Autodesk Inventor part; units mm, degrees
ref_plane "YZ Plane" through (0, 0, 0) normal (1, 0, 0) x (0, 1, 0)
ref_plane "XZ Plane" through (0, 0, 0) normal (0, 1, 0) x (-1, 0, 0)
ref_plane "XY Plane" through (0, 0, 0) normal (0, 0, 1) x (1, 0, 0)
sketch "Sketch1" plane through (0, 0, 0) normal (0, 0, 1) x (1, 0, 0)
  line L0 (-7.5896, 2.5423) -> (-6.4349, 4.5423)
  line L1 (-6.4349, 4.5423) -> (-4.1255, 4.5423)
  line L2 (-4.1255, 4.5423) -> (-2.9708, 2.5423)
  line L3 (-2.9708, 2.5423) -> (-4.1255, 0.5423)
  line L4 (-4.1255, 0.5423) -> (-6.4349, 0.5423)
  line L5 (-6.4349, 0.5423) -> (-7.5896, 2.5423)
  circle A0 centre (-5.2802, 2.5423) radius 1
  dimension "d0" = 4
  dimension "d1" = 2
extrude "Extrusion1" add sketch "Sketch1" along normal blind 10 contours L0 L1 L2 L3 L4 L5 | A0
extrude "Extrusion2" add sketch "Sketch1" against normal blind 6 contours A0
sketch "Sketch2" plane through (0, 0, 10) normal (0, 0, 1) x (1, 0, 0)
  circle A0 centre (-5.2802, 2.5423) radius 1
  circle A1 centre (-5.2802, 2.5423) radius 1.5
  point P0 (0, 0)
hole "Hole1" at (-5.2802, 2.5423, 10) direction (0, 0, -1) diameter 2 depth 7 tip angle 120
chamfer "Chamfer1" distance 0.1 angle 45 1 edges at (-6.2802, 2.5423, -6)
thread "Thread3"
thread "Thread4"
properties part number "Espaciador de Plástico M2 L10" material "Brass, Soft Yellow"
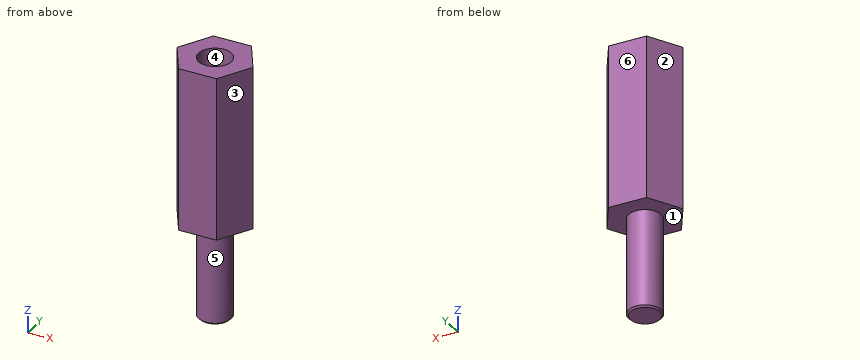
Input: part model. Units: mm. Frame: model coordinates. Face numbers are marked on the shaded views. A direction names the side the tool comes from. Round coordinates to 2 decimals unless told otherwise and drop trailing zeros. Loops run counter-clockwise (first coordinate to the right, second up) from the corner with the lowest first, then second, coordinate; pieces in that order, holes last.
1) Pin query (flat end, axial travel): pin 1 (1.5 mm diameter, centred on y = 3.5, z = 4, fed in from -X); pin 2 (1 mm diameter, centred on x = -3.5, y = 1.5, fed in from -Z). Return the tip coordinate at first contact, or that it passes through.
Ans:
pin 1: stops at x = -7.47
pin 2: stops at z = 0
2) Pull-direction query (Y, two-part tool) for the marked faces 3, 4, 5 and 6; classes: released by +Y, released by -Y, zero draft, split by the parting line, or undercut.
Ans:
face 3: released by -Y
face 4: undercut
face 5: split by the parting line
face 6: released by +Y
3) Section query A-A on z = 3.75. Return the cut outline in (x, y), plus the area to 3 significant figures.
Ans:
outline: (-7.59, 2.54) - (-6.43, 0.54) - (-4.13, 0.54) - (-2.97, 2.54) - (-4.13, 4.54) - (-6.43, 4.54) - close; hole circle Ø2 at (-5.28, 2.54)
area: 10.7 mm2
4) Material intervals for line 1 (Z direction, x = -3.9, y = 3.55); line 2 (Y direction, x = -4.5, z = 3.5); line 3 (Y direction, x = -4.6, z = 5.75), sorted ascending.
Ans:
line 1: z = 0 to 10
line 2: y = 0.54 to 1.92, 3.17 to 4.54
line 3: y = 0.54 to 1.81, 3.28 to 4.54
5) Set-up query: the marked faces 1 and 2. Return all of +Z, -Z, +X, -X, +Y, -Y with unobstructed straight access to the full face (end or side cutting, diameter ignored); none if empty.
Ans:
face 1: -Z
face 2: +Z, -Z, -X, +Y
6) Section query D-D on x = -6.95. Return the cut outline in (y, z).
Ans:
outline: (1.43, 0) - (3.65, 0) - (3.65, 10) - (1.43, 10) - close
7) Section query C-C on y = 1. Return the cut outline in (x, z).
Ans:
outline: (-6.7, 0) - (-3.86, 0) - (-3.86, 10) - (-6.7, 10) - close
8) Section query B-B on z = 1. Return the cut outline in (x, y).
Ans:
outline: (-7.59, 2.54) - (-6.43, 0.54) - (-4.13, 0.54) - (-2.97, 2.54) - (-4.13, 4.54) - (-6.43, 4.54) - close
